Verification items for the finished model (mm, model axes). A direction names the side the tool comes from. Coordinates: 2 decimals unless noted, no trailing zeros. Order: outer loops, then holes, each group sorted by start corner. A loop starts at its lowest first (then second) coordinate and runs counter-clockwise, first axis right, second up. Notation, with made-up numbers: M 33,-36 L 92,-36 A19 ccw 92,-7 Z; hole C -14.75,-11 d7. An arc over 180 degrees is marked long. Return JSON: item names as keys, results as strings. Group by question number.
Q1. Thickness scan on probe 1 along X at (y, z) = (2, -75); probe 2 along Y at (x, z) = (11, -25.5); probe 3 along X at (y, z) = (99, -30). Record the ranges inside material, lowest first.
Q2. Section check A-A, the plane y = 25.5. Enter the section's corners in (x, z).
Q3. Section check B-B, the plane x = 22. Enter the section's corners in (y, z), then the cut area to 3 significant figures.
Q4. Mould release check, pull along Y, two halves, no side actions. Record for faces 1 (the face through (20.11, 64.198, -29.373)), 2 (the face through (20.11, 78.94, -22.326)), 3 (the face through (34.425, 1.972, -73.614)): pulls with the +Y half, pulls with the -Y half, needs draft (parallel to the pull), parting line crosses it, or undercut.
Q5. Section check D-D, the plane z = -31. Enter the section's corners in (x, y), then the cut area to 3 significant figures.
Q6. Go/stop test with flat-tipped pins: pin 1 Ø2 at (x, y) = (20.5, 140) entering from +Z; pin 2 Ø6 at (x, y) = (19.5, 105) entering from -Z; pin 3 Ø8 at (x, z) = (19, -24) entering from -Y; pin 4 Ø4 at (x, y) = (26, 32.5) entering from +Z. Record where each tip stops, or that it passes through.
Q7. Section check C-C, the plane z = -66. Enter the section's corners in (x, y), then the cut area to 3 significant figures.
Q8. Access from +Z, -Z, +X, -X, +Y, -Y to the whole of each face (thin tool, end or side, straight path). Record for faces 4 (the face through (27.85, 74, -51)), 5 (the face through (12.15, 74, -51)), 6 (the face through (38, 2, -79)), 7 (the face through (20.11, 65.91, -50.36)), 8 (the face through (1, 2, -78)).
from build123d import *

# Parameters (mm, degrees)
SKETCH1_W           = 40
SKETCH1_H           = 80
SKETCH1_R           = 1.54
SKETCH1_R_2         = 1.5
BOSS_EXTRUDE1_DEPTH = 4
FILLET1_R           = 5
SKETCH2_W           = 15.7
SKETCH2_H           = 60
BOSS_EXTRUDE2_DEPTH = 152
SKETCH3_R           = 3
CUT_EXTRUDE1_DEPTH  = 160
CUT_EXTRUDE2_DEPTH  = 160
FILLET2_R           = 5
CUT_EXTRUDE3_DEPTH  = 160
FILLET3_R           = 1


with BuildPart() as part:
    # Sketch1 → Boss-Extrude1 (new body)
    with BuildSketch(Plane(origin=(0, 0, 0), x_dir=(1, 0, 0), z_dir=(0, 1, 0))):
        with Locations((20, 40)):
            Rectangle(SKETCH1_W, SKETCH1_H)
        with Locations(Location((5, 75, 0), (0, 0, 270))):
            Circle(SKETCH1_R, mode=Mode.SUBTRACT)
        with Locations(Location((35, 75, 0), (0, 0, 270))):
            Circle(SKETCH1_R_2, mode=Mode.SUBTRACT)
        with Locations(Location((5, 5, 0), (0, 0, 270))):
            Circle(SKETCH1_R_2, mode=Mode.SUBTRACT)
        with Locations(Location((35, 5, 0), (0, 0, 270))):
            Circle(SKETCH1_R_2, mode=Mode.SUBTRACT)
    extrude(amount=BOSS_EXTRUDE1_DEPTH)

    # Fillet1
    fillet1_edges = [part.edges().sort_by_distance(p)[0] for p in [
        (0, 2, -80),
        (40, 2, -80),
        (40, 2, 0),
        (0, 2, 0),
    ]]
    fillet(fillet1_edges, radius=FILLET1_R)

    # Sketch2 → Boss-Extrude2 (add)
    with BuildSketch(Plane(origin=(0, 4, 0), x_dir=(1, 0, 0), z_dir=(0, 1, 0))):
        with Locations((20, 40)):
            Rectangle(SKETCH2_W, SKETCH2_H)
    extrude(amount=BOSS_EXTRUDE2_DEPTH)

    # Sketch3 → Cut-Extrude1 (cut)
    with BuildSketch(Plane(origin=(40, 0, 0), x_dir=(0, 0, -1), z_dir=(1, 0, 0))):
        with Locations((40, 150)):
            Circle(SKETCH3_R)
    extrude(amount=-CUT_EXTRUDE1_DEPTH, mode=Mode.SUBTRACT)

    # Sketch4 → Cut-Extrude2 (cut)
    with BuildSketch(Plane(origin=(40, 0, 0), x_dir=(0, 0, -1), z_dir=(1, 0, 0))):
        Polygon((35, 156), (10, 4), (10, 156), align=None)
        Polygon((45, 156), (70, 4), (70, 156), align=None)
    extrude(amount=-CUT_EXTRUDE2_DEPTH, mode=Mode.SUBTRACT)

    # Fillet2
    fillet2_edges = [part.edges().sort_by_distance(p)[0] for p in [
        (20, 156, -45),
        (20, 156, -35),
    ]]
    fillet(fillet2_edges, radius=FILLET2_R)

    # Sketch5 → Cut-Extrude3 (cut)
    with BuildSketch(Plane(origin=(27.85, 0, 0), x_dir=(0, 0, -1), z_dir=(1, 0, 0))):
        Polygon((20, 4), (40, 132.452325787), (60, 4), align=None)
    extrude(amount=-CUT_EXTRUDE3_DEPTH, mode=Mode.SUBTRACT)

    # Fillet3
    fillet3_edges = [part.edges().sort_by_distance(p)[0] for p in [
        (20, 132.452325787, -40),
    ]]
    fillet(fillet3_edges, radius=FILLET3_R)


solid = part.part
Numbers:
{
 "1": {"probe 1": "x = 0 to 3.46, 6.54 to 33.5, 36.5 to 40", "probe 2": "y = 0 to 4", "probe 3": "x = 12.15 to 27.85"},
 "2": {"outline": "M 12.15,-66.46 L 27.85,-66.46 L 27.85,-56.65 L 12.15,-56.65 Z; M 12.15,-23.35 L 27.85,-23.35 L 27.85,-13.54 L 12.15,-13.54 Z"},
 "3": {"outline": "M 0,-80 L 4,-80 L 4,-70 L 151.81,-45.69 A5 ccw 156,-40.76 L 156,-39.24 A5 ccw 151.81,-34.31 L 4,-10 L 4,0 L 0,0 Z; hole M 4,-60 L 126.11,-40.99 A1 ccw 126.11,-39.01 L 4,-20 Z; hole C 150,-40 d6", "area": "3,040 mm2"},
 "4": {"face 1": "undercut", "face 2": "pulls with the +Y half", "face 3": "needs draft"},
 "5": {"outline": "M 0,0 L 40,0 L 40,4 L 0,4 Z; M 12.15,74.65 L 27.85,74.65 L 27.85,131.68 L 12.15,131.68 Z", "area": "1,060 mm2"},
 "6": {"pin 1": "stops at z = -32.2", "pin 2": "stops at z = -53.88", "pin 3": "stops at y = 0", "pin 4": "stops at z = -14.36"},
 "7": {"outline": "M 0,0 L 40,0 L 40,4 L 27.85,4 L 27.85,28.32 L 12.15,28.32 L 12.15,4 L 0,4 Z", "area": "542 mm2"},
 "8": {"face 4": "+Z, -Z, +X, +Y", "face 5": "+Z, -Z, -X, +Y", "face 6": "-Z, +X, +Y, -Y", "face 7": "+X, -X", "face 8": "-Z, -X, +Y, -Y"}
}
